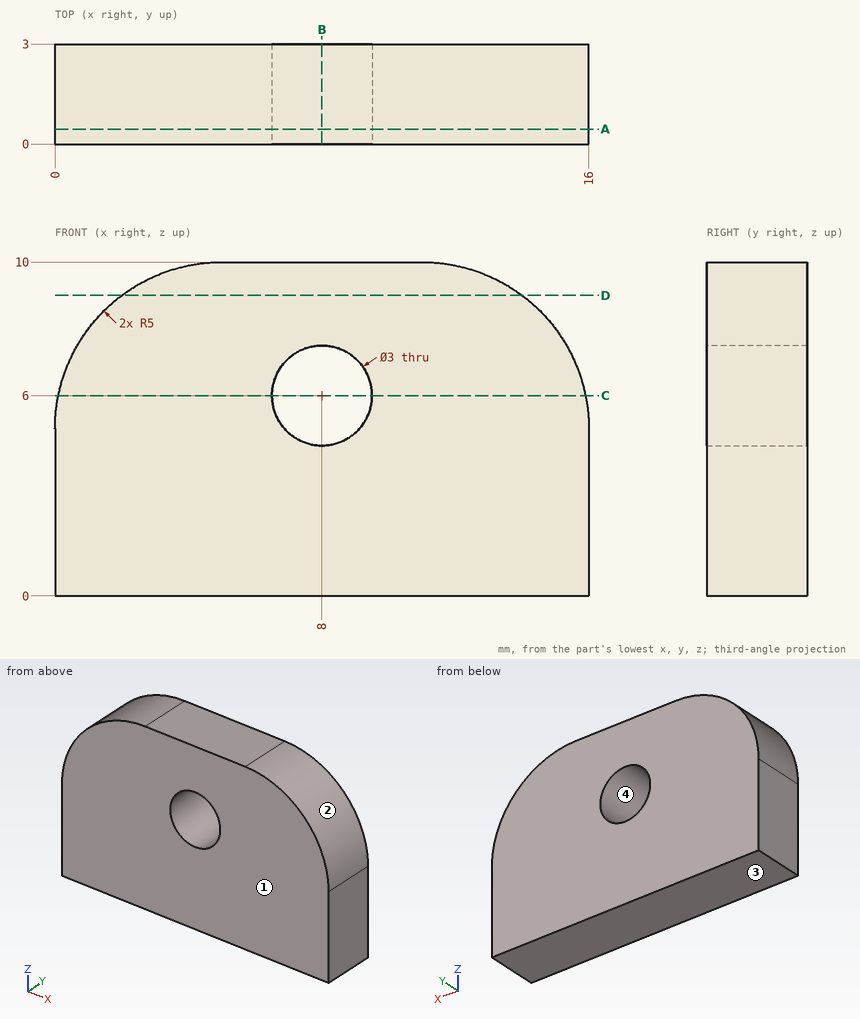
Geometry check sheet. Reference: drawing and pictorial views, mm from the part's lowest x, y, z. Round coordinates to 2 decimals unless told otherwise and drop trailing zeros. Order: outer loops, then holes, each group sorted by start corner. A loop starts at its lowest first (then second) coordinate and runs counter-clockwise, first axis right, second up.
Q1. Cross-section at D-D, the plane z = 9. Enter the section's corners in (x, y).
Filled sheet:
outline: (2, 0) - (14, 0) - (14, 3) - (2, 3) - close
Q2. Depth check by flat-ended pin: P1, Ø2.5, axis at x = 8, z = 6, coming from the +Y side. Enter the tip coordinate at first touch or a pass-through.
Filled sheet:
P1: passes through
Q3. Cross-section at B-B, the plane x = 8. Enter the section's corners in (y, z).
Filled sheet:
outline: (0, 0) - (3, 0) - (3, 4.5) - (0, 4.5) - close; (0, 7.5) - (3, 7.5) - (3, 10) - (0, 10) - close
Q4. Scan lines: L1, parallel to Z at x = 8, y = 1.55; L2, parallel to X at y = 1.25, z = 6; L3, parallel to X at y = 0.4, z = 6.25. Record each from-to range of solid material in increasing order.
Filled sheet:
L1: z = 0 to 4.5, 7.5 to 10
L2: x = 0.1 to 6.5, 9.5 to 15.9
L3: x = 0.16 to 6.52, 9.48 to 15.84
Q5. Cross-section at A-A, the plane y = 0.45. Enter the section's corners in (x, z).
Filled sheet:
outline: (0, 0) - (16, 0) - (16, 5) arc R5 ccw to (11, 10) - (5, 10) arc R5 ccw to (0, 5) - close; hole circle Ø3 at (8, 6)
Q6. Draft check along Z on the marked faces 1, 2, 3 and 4. Enter one of: pulls with the +Z half, pulls with the -Z half, needs draft (parallel to the pull), parting line crosses it, or undercut.
Filled sheet:
face 1: needs draft
face 2: pulls with the +Z half
face 3: pulls with the -Z half
face 4: undercut
Q7. Cross-section at C-C, the plane z = 6. Enter the section's corners in (x, y), plus the area to 3 significant figures.
Filled sheet:
outline: (0.1, 0) - (6.5, 0) - (6.5, 3) - (0.1, 3) - close; (9.5, 0) - (15.9, 0) - (15.9, 3) - (9.5, 3) - close
area: 38.4 mm2
